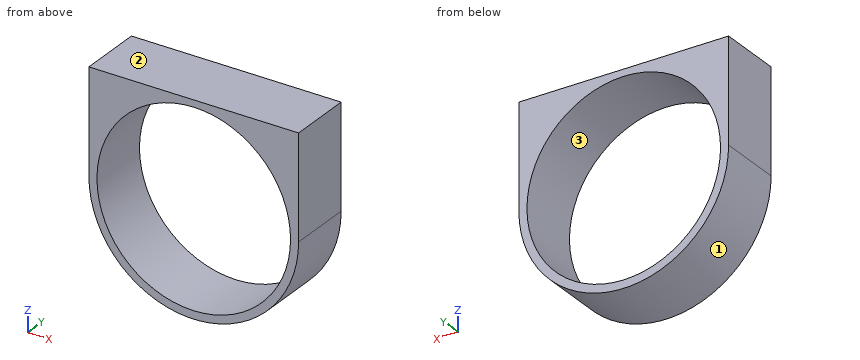
from build123d import *

# Parameters (mm, degrees)
SKETCH1_R           = 3
BOSS_EXTRUDE1_DEPTH = 2


with BuildPart() as part:
    # Sketch1 → Boss-Extrude1 (new body)
    with BuildSketch(Plane(origin=(0, 0, 0), x_dir=(1, 0, 0), z_dir=(0, 1, 0))):
        with BuildLine():
            Line((-3.25, 0), (-3.25, -3.213400023))
            Line((-3.25, -3.213400023), (0.25, -3.213400023))
            Line((0.25, -3.213400023), (3.25, -3.213400023))
            Line((3.25, -3.213400023), (3.25, 0))
            ThreePointArc((3.25, 0), (0, 3.25), (-3.25, 0))
        make_face()
        with Locations(Location((0, 0, 0), (0, 0, 270))):
            Circle(SKETCH1_R, mode=Mode.SUBTRACT)
    extrude(amount=BOSS_EXTRUDE1_DEPTH)


solid = part.part
Can you work these out from the model? Positions are in its coordinate system, mm. Face numbers are marked on the shaded views. Give positions to 0.01 mm unless a question says otherwise; leave off trailing zeros. Order: outer loops, then holes, each group sorted by start corner. A loop starts at its lowest first (then second) coordinate and runs counter-clockwise, first axis right, second up. Notation, with made-up numbers: M 85.5,37 L 130.5,37 A35 ccw 130.5,71 Z; hole C 50.5,-32 d4. An arc over 180 degrees is marked long. Use a Markdown table: item, result. Add a question column.
Item 1: Suppose I cut it at C-C (y = 1.25). List the corners of the cut face in (x, z) for me, then the cut area to 3 significant figures.
Item 2: If I drill on L1, parallel to X at y = 0.9, z = 0; L2, parallel to X at y = 0.55, z = -2.75; L3, parallel to Z at x = 1.75, y = 1.25, over which ranges is the centre line in solid material (lowest first)? Write a range as [from, to].
Item 3: Suppose I cut it at B-B (z = -1). List the corners of the cut face in (x, y) for me, then the cut area to 3 significant figures.
Item 4: Suppose I cut it at A-A (x = 0). List the corners of the cut face in (y, z) for me, then the cut area to 3 significant figures.
Item 5: We'd pull the mould along X, two halves only. Please class the marked faces 1, 2 and 3: +X half, -X half, draft (parallel to the pull), parting line (faces both ways), or undercut.
Answer sheet:
| question | item | result |
|---|---|---|
| 1 | outline | M -3.25,0 A3.25 ccw 3.25,0 L 3.25,3.21 L -3.25,3.21 Z; hole C 0,0 d6 |
| 1 | area | 9.20 mm² |
| 2 | L1 | x = [-3.25, -3], [3, 3.25] |
| 2 | L2 | x = [-1.73, -1.2], [1.2, 1.73] |
| 2 | L3 | z = [-2.74, -2.44], [2.44, 3.21] |
| 3 | outline | M -3.09,0 L -2.83,0 L -2.83,2 L -3.09,2 Z; M 2.83,0 L 3.09,0 L 3.09,2 L 2.83,2 Z |
| 3 | area | 1.06 mm² |
| 4 | outline | M 0,-3.25 L 2,-3.25 L 2,-3 L 0,-3 Z; M 0,3 L 2,3 L 2,3.21 L 0,3.21 Z |
| 4 | area | 0.927 mm² |
| 5 | face 1 | parting line |
| 5 | face 2 | draft |
| 5 | face 3 | undercut |
